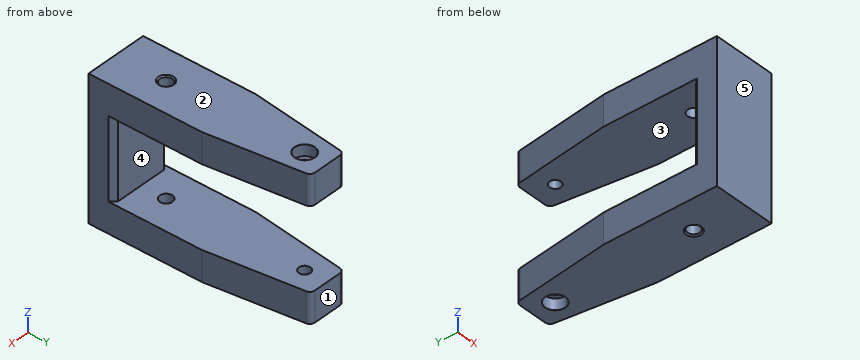
from build123d import *

# Parameters (mm, degrees)
BOSS_EXTRUDE1_DEPTH = 28
SKETCH2_W           = 32
SKETCH2_H           = 74
CUT_EXTRUDE1_DEPTH  = 93.005434622
CHAMFER1_SIZE       = 2
FILLET1_R           = 2


with BuildPart() as part:
    # Sketch1 → Boss-Extrude1 (new, symmetric)
    with BuildSketch(Plane.XY):
        Polygon((12.5, 0), (-12.5, 0), (-12.5, 45), (-7.5, 84), (7.5, 84), (12.5, 45), align=None)
    extrude(amount=BOSS_EXTRUDE1_DEPTH, both=True)

    # Sketch2 → Cut-Extrude1 (cut, through all)
    with BuildSketch(Plane(origin=(12.5, 0, 0), x_dir=(0, 0, -1), z_dir=(1, 0, 0))):
        with Locations((0, 47)):
            Rectangle(SKETCH2_W, SKETCH2_H)
    extrude(amount=-CUT_EXTRUDE1_DEPTH, mode=Mode.SUBTRACT)

    # Sketch7 → CBORE for M4 Hex Socket Head Cap Screw1 (revolve, cut)
    with BuildSketch(Plane(origin=(0, 75, 28), x_dir=(0, -1, 0), z_dir=(1, 0, 0))):
        Polygon((0, 0), (0, 21.351936393), (2.25, 20), (2.25, 4.4), (4, 4.4), (4, 0.025), (4.025, 0), align=None)
    cbore_for_m4_hex_socket_head_cap_screw1 = revolve(axis=Axis((0, 75, 34.35), (0, 0, -1)), mode=Mode.SUBTRACT)

    # Mirror1: CBORE for M4 Hex Socket Head Cap Screw1 across plane
    add(cbore_for_m4_hex_socket_head_cap_screw1.mirror(Plane.XY), mode=Mode.SUBTRACT)

    # Sketch9 → M6 Tapped Hole1 (revolve, cut)
    with BuildSketch(Plane(origin=(0, 20, 28), x_dir=(0, -1, 0), z_dir=(1, 0, 0))):
        Polygon((0, 0), (0, 28.502151548), (2.5, 27), (2.5, 0.525), (3.025, 0), align=None)
    m6_tapped_hole1 = revolve(axis=Axis((0, 20, 34.35), (0, 0, -1)), mode=Mode.SUBTRACT)

    # Chamfer1
    chamfer1_edges = [part.edges().sort_by_distance(p)[0] for p in [
        (12.5, 10, 0),
        (-12.5, 10, 0),
    ]]
    chamfer(chamfer1_edges, length=CHAMFER1_SIZE)

    # Fillet1
    fillet1_edges = [part.edges().sort_by_distance(p)[0] for p in [
        (-7.5, 84, 22),
        (7.5, 84, 22),
        (-7.5, 84, -22),
        (7.5, 84, -22),
    ]]
    fillet(fillet1_edges, radius=FILLET1_R)

    # Mirror2: M6 Tapped Hole1 across plane
    add(m6_tapped_hole1.mirror(Plane.XY), mode=Mode.SUBTRACT)


solid = part.part
Geometry: final body of the model. Coordinates: model frame, mm. Face numbers are marked on the shaded views. A direction names the side the tool comes from. Coordinates: 2 decimals unless noted, no trailing zeros. Order: outer loops, then holes, each group sorted by start corner. A loop starts at its lowest first (then second) coordinate and runs counter-clockwise, first axis right, second up. Notation, with made-up numbers: (24.25, 50) - (52.25, 50) arc R19 cw to (52.25, 76) - close; hole circle Ø5 at (-25, 46.25). An arc over 180 degrees is marked (long way). Use one line per item in the form item = value.
1) Section D-D (x = 9.25). Return loops of the section in (y, z).
Solutions:
outline = (0, -28) - (70.35, -28) - (70.35, -16) - (10, -16) - (10, 16) - (70.35, 16) - (70.35, 28) - (0, 28) - close
2) Ray query, L1, parallel to Y at x = 0, z = 18.5; L2, parallel to Y at x = 0, z = -26.35; L3, parallel to Z at x = -4.25, y = 42.5. Return the intervals inside material, ascending.
Solutions:
L1 = 0 to 17.5, 22.5 to 72.75, 77.25 to 84
L2 = 0 to 17.5, 22.5 to 71, 79 to 84
L3 = -28 to -16, 16 to 28
3) Section A-A (y = 42). Return loops of the section in (x, z).
Solutions:
outline = (-12.5, -28) - (12.5, -28) - (12.5, -16) - (-12.5, -16) - close; (-12.5, 16) - (12.5, 16) - (12.5, 28) - (-12.5, 28) - close
4) Section B-B (z = 22). Return loops of the section in (x, y).
Solutions:
outline = (-12.5, 0) - (12.5, 0) - (12.5, 45) - (7.72, 82.25) arc R2 ccw to (5.74, 84) - (-5.74, 84) arc R2 ccw to (-7.72, 82.25) - (-12.5, 45) - close; hole circle Ø5 at (0, 20); hole circle Ø4.5 at (0, 75)
5) Section C-C (y = 20). Return loops of the section in (x, z) (3 decimals).
Solutions:
outline = (-12.5, -28) - (-3.025, -28) - (-2.5, -27.475) - (-2.5, -16) - (-12.5, -16) - close; (-12.5, 16) - (-2.5, 16) - (-2.5, 27.475) - (-3.025, 28) - (-12.5, 28) - close; (2.5, -27.475) - (3.025, -28) - (12.5, -28) - (12.5, -16) - (2.5, -16) - close; (2.5, 16) - (12.5, 16) - (12.5, 28) - (3.025, 28) - (2.5, 27.475) - close
6) Set-up query: the marked faces 4 and 5. Return all of +Z, -Z, +X, -X, +Y, -Y with unobstructed straight access to the full face (end or side cutting, diameter ignored); none if empty.
Solutions:
face_4 = +X, -X, +Y
face_5 = +Z, -Z, +X, -X, -Y
7) Mould query, pull axis Z, two halves, no side actions, for the marked faces 1, 2 and 3. Classes: +Z half, -Z half, draft (parallel to the pull), parting line (faces both ways), or undercut.
Solutions:
face_1 = draft
face_2 = +Z half
face_3 = undercut
8) Pin query (flat end, axial travel): pin 1 (6 mm diameter, centred on x = 0, y = 75, fed in from -Z); pin 2 (6 mm diameter, centred on x = 0, y = 20, fed in from -Z) (3 decimals); pin 3 (4 mm diameter, centred on x = 1.5, y = 74.5, fed in from +Z); pin 4 (4 mm diameter, centred on x = -3, z = 7.5, fed in from -Y). Return the tip coordinate at first contact, or that it passes through.
Solutions:
pin_1 = -23.6
pin_2 = -27.975
pin_3 = 23.6
pin_4 = 0
